```python
from build123d import *

# Parameters (mm, degrees)
F0_W     = 120
F0_H     = 120
F1_DEPTH = 246.38
F2_W     = 120
F2_H     = 120
F2_W_2   = 96
F2_H_2   = 96
F3_DEPTH = 39
F4_R     = 105
F4_W     = 120
F4_H     = 120
F5_DEPTH = 100
F7_DEPTH = 80


# Not quite as in the source:
# - a fillet or chamfer that OpenCascade refuses, or shapes differently, is made with other operations: its cross-section is extruded or revolved along the edge and cut away or added


with BuildPart() as f1:
    # F0 (on Top) → F1 (new body)
    with BuildSketch(Plane.XY):
        with Locations((60, 60)):
            Rectangle(F0_W, F0_H)
    extrude(amount=F1_DEPTH)

    # F2 (on face) → F3 (cut)
    with BuildSketch(Plane.XY.offset(246.38)):
        with Locations((60, 60)):
            Rectangle(F2_W, F2_H)
        with Locations((60, 60)):
            Rectangle(F2_W_2, F2_H_2, mode=Mode.SUBTRACT)
    extrude(amount=-F3_DEPTH, mode=Mode.SUBTRACT)

    # F4 (on face) → F5 (join)
    with BuildSketch(Plane(origin=(0, 0, 0), x_dir=(1, 0, 0), z_dir=(0, 0, -1))):
        with Locations((60, -60)):
            Circle(F4_R)
        with Locations((60, -60)):
            Rectangle(F4_W, F4_H, mode=Mode.SUBTRACT)
    extrude(amount=-F5_DEPTH)

    # F6: chamfer of 70 on 1 edges, made by hand


with BuildPart() as f6_tool2:
    # F6_s3 → F6_t4 (revolve)
    with BuildSketch(Plane.XZ.offset(-60)):
        Polygon((95, 100), (165, 30), (165, 100), align=None)
    revolve(axis=Axis((60, 60, 100), (0, 0, -1)))

    split(bisect_by=Plane.YZ.offset(120), keep=Keep.TOP)


with BuildPart() as f1_1:
    add(f1.part)

    # F6_t1: cut F6_tool2
    add(f6_tool2.part, mode=Mode.SUBTRACT)


with BuildPart() as f6_tool7:
    # F6_s8 → F6_t9 (revolve)
    with BuildSketch(Plane.XZ.offset(-60)):
        Polygon((95, 100), (165, 30), (165, 100), align=None)
    revolve(axis=Axis((60, 60, 100), (0, 0, -1)))

    split(bisect_by=Plane.XZ, keep=Keep.TOP)


with BuildPart() as f1_2:
    add(f1_1.part)

    # F6_t6: cut F6_tool7
    add(f6_tool7.part, mode=Mode.SUBTRACT)


with BuildPart() as f6_tool12:
    # F6_s13 → F6_t14 (revolve)
    with BuildSketch(Plane.XZ.offset(-60)):
        Polygon((95, 100), (165, 30), (165, 100), align=None)
    revolve(axis=Axis((60, 60, 100), (0, 0, -1)))

    split(bisect_by=Plane.YZ, keep=Keep.BOTTOM)


with BuildPart() as f1_3:
    add(f1_2.part)

    # F6_t11: cut F6_tool12
    add(f6_tool12.part, mode=Mode.SUBTRACT)


with BuildPart() as f6_tool17:
    # F6_s18 → F6_t19 (revolve)
    with BuildSketch(Plane.XZ.offset(-60)):
        Polygon((95, 100), (165, 30), (165, 100), align=None)
    revolve(axis=Axis((60, 60, 100), (0, 0, -1)))

    split(bisect_by=Plane.XZ.offset(-120), keep=Keep.BOTTOM)


with BuildPart() as f1_4:
    add(f1_3.part)

    # F6_t16: cut F6_tool17
    add(f6_tool17.part, mode=Mode.SUBTRACT)


with BuildPart() as f7:
    # F7 (new): a face of the model
    f7_faces = [f1_4.part.faces().sort_by_distance(p)[0] for p in [
        (60, 118.3029437252, 207.38),
    ]]
    extrude(f7_faces, amount=F7_DEPTH)


solid = f1_4.part
```
Verification items for the finished model (mm, model axes). A direction names the side the tool comes from. Give positions to 0.01 mm unless a question says otherwise; leave off trailing zeros. Order: outer loops, then holes, each group sorted by start corner. A loop starts at its lowest first (then second) coordinate and runs counter-clockwise, first axis right, second up. Notation, with made-up numbers: M 35.5,9 L 43.5,9 A19 cw 43.5,26 Z; hole C 70.5,-34 d9. An arc over 180 degrees is marked long. Answer in a Markdown table with one row per item. Add a question column.
Item 1: Gauge pin test, flat ends, axial feed: pin 1 (5 mm diameter, centred on y = 129.5, z = 42.5, fed in from +X); pin 2 (4 mm diameter, centred on x = 8.5, y = 85.5, fed in from -Z); pin 3 (2 mm diameter, centred on x = 94.5, z = 155.5, fed in from +Y); pin 4 (11.5 mm diameter, centred on x = 58, z = 229.5, fed in from -Y). Record the tip position at first contact, or that the pin passes through.
Item 2: Section check D-D, the plane z = 214.5. Enter the section's corners in (x, y).
Item 3: Scan lines: probe 1 along X at (y, z) = (2.5, 114.5); probe 2 along Y at (x, z) = (89.5, 210). Record each from-to range of solid material in increasing order. Write a range as from..to.
Item 4: Tool access check on faces 1 (the flat face through (12, 59, 227)), 2 (the flat face through (59, 12, 227)), 3 (the flat face through (108, 59, 227)). Record the directions out of +Z, -Z, +X, -X, +Y, -Y that give a thin tool (end or side, any length) a straight path to the whole face; none if there is none.
Item 5: Section check C-C, the plane z = 189.5. Enter the section's corners in (x, y).
Item 6: Section check A-A, the plane y = 60. Enter the section's corners in (x, z).
Filled sheet:
| question | item | result |
|---|---|---|
| 1 | pin 1 | stops at x = 125.62 |
| 1 | pin 2 | stops at z = 0 |
| 1 | pin 3 | stops at y = 120 |
| 1 | pin 4 | stops at y = 12 |
| 2 | outline | M 12,12 L 108,12 L 108,108 L 12,108 Z |
| 3 | probe 1 | x = 0..120 |
| 3 | probe 2 | y = 12..108 |
| 4 | face 1 | +Z, -X, +Y, -Y |
| 4 | face 2 | +Z, +X, -X, -Y |
| 4 | face 3 | +Z, +X, +Y, -Y |
| 5 | outline | M 0,0 L 120,0 L 120,120 L 0,120 Z |
| 6 | outline | M -45,0 L 165,0 L 165,30 L 120,75 L 120,207.38 L 108,207.38 L 108,246.38 L 12,246.38 L 12,207.38 L 0,207.38 L 0,75 L -45,30 Z |
